Design review of the part built by this model. Coordinates are the model's own, in mm. A direction names the side the tool comes from. Give positions to 0.01 mm unless a question says otherwise; leave off trailing zeros. Order: outer loops, then holes, each group sorted by start corner. A loop starts at its lowest first (then second) coordinate and runs counter-clockwise, first axis right, second up. Notation, with made-up numbers: (12, -21.5) -> (71, -21.5) arc R18 cw to (71, -9.5) -> close; hole circle Ø7 at (6, 38). An arc over 180 degrees is marked (long way). Answer in a Markdown table with one row per item. Add a question column.
```python
from build123d import *

# Parameters (mm, degrees)
BOSS_EXTRUDE2_DEPTH      = 25
BOSS_EXTRUDE2_DEPTH_BACK = 150
SKETCH3_R                = 35
SKETCH4_R                = 35
SKETCH4_R_2              = 15
CUT_EXTRUDE1_DEPTH       = 40
CUT_EXTRUDE2_START       = -80
CUT_EXTRUDE2_DEPTH       = 80
SKETCH7_R                = 15
CUT_EXTRUDE3_DEPTH       = 164.554272338


with BuildPart() as part:
    # Sketch3 → Boss-Extrude2 (new, two sides: drawn at the far end of the back side and taken through both)
    with BuildSketch(Plane.XY.offset(-BOSS_EXTRUDE2_DEPTH_BACK)):
        Circle(SKETCH3_R)
    extrude(amount=BOSS_EXTRUDE2_DEPTH + BOSS_EXTRUDE2_DEPTH_BACK)

    # Sketch4 → Cut-Extrude1 (cut)
    with BuildSketch(Plane(origin=(0, 0, -150), x_dir=(-1, 0, 0), z_dir=(0, 0, -1))):
        Circle(SKETCH4_R)
        Circle(SKETCH4_R_2, mode=Mode.SUBTRACT)
    extrude(amount=-CUT_EXTRUDE1_DEPTH, mode=Mode.SUBTRACT)

    # Sketch5 → Cut-Extrude2 (cut)
    with BuildSketch(Plane.XY.offset(25).offset(CUT_EXTRUDE2_START)):
        with BuildLine():
            Line((-28.722813233, 20), (28.722813233, 20))
            ThreePointArc((28.722813233, 20), (0, 35), (-28.722813233, 20))
        make_face()
        with BuildLine():
            Line((-28.722813233, -20), (28.722813233, -20))
            ThreePointArc((28.722813233, -20), (0, -35), (-28.722813233, -20))
        make_face()
    extrude(amount=CUT_EXTRUDE2_DEPTH, mode=Mode.SUBTRACT)

    # Sketch7 → Cut-Extrude3 (cut, through all)
    with BuildSketch(Plane.XZ.offset(20)):
        with Locations(Location((0, 0, 0), (0, 0, 270))):
            Circle(SKETCH7_R)
    extrude(amount=-CUT_EXTRUDE3_DEPTH, mode=Mode.SUBTRACT)


solid = part.part
```
1) Clearance check with flat-ended pins moving along their axes: P1, Ø2, axis at y = -5.5, z = -25, coming from the +X side; P2, Ø7.5, axis at x = 2.5, y = -30.5, coming from the +Z side; P3, Ø1, axis at y = -19.5, z = -96, coming from the +X side. State where each tip first meets the part, or that it passes through.
2) For L1, parallel to Y at x = 0.5, z = -90; L2, parallel to Y at x = 22.5, z = -49; L3, parallel to Z at x = 30.5, y = -17, list the stretches that pass through material, from the lowest coordinate up.
3) Add section B-B, the plane z = 0. Write out the cut boundary in (x, y).
4) Mouldability with a two-part tool opening along X and no side actions: class faces 4 (the face through (0.66, -0.28, 14.985)), 5 (the face through (33.384, 10.513, -58.445)), 6 (the face through (-15, -7, -110)) as +X half, -X half, draft (parallel to the pull), parting line (faces both ways), or undercut.
5) Add section D-D, the plane y = 0. Write out the cut boundary in (x, z).
6) Machinability: for faces 1 (the face through (0, -26, -55)), 2 (the face through (14.985, 0.66, -130.28)), 3 (the face through (0, 20, -16)), which of the approach directions +Z, -Z, +X, -X, +Y, -Y give a long, thin tool a straight path to every point of the face, cutting with its end or side? Answer none if there is none.
7) Add section C-C, the plane x = -21. Write out the cut boundary in (y, z), and give its area (3 significant figures).
8) Add section A-A, the plane x = 0. Write out the cut boundary in (y, z), and give its area (3 significant figures).
Verdict:
| question | item | result |
|---|---|---|
| 1 | P1 | stops at x = 34.71 |
| 1 | P2 | stops at z = -55 |
| 1 | P3 | stops at x = 29.39 |
| 2 | L1 | y = -35 to 35 |
| 2 | L2 | y = -20 to 20 |
| 2 | L3 | z = -110 to 25 |
| 3 | outline | (-28.72, -20) -> (-15, -20) -> (-15, 20) -> (-28.72, 20) arc R35 ccw to start; (15, -20) -> (28.72, -20) arc R35 ccw to (28.72, 20) -> (15, 20) -> close |
| 4 | face 4 | undercut |
| 4 | face 5 | parting line |
| 4 | face 6 | draft |
| 5 | outline | (-35, -110) -> (-15, -110) -> (-15, -150) -> (15, -150) -> (15, -110) -> (35, -110) -> (35, 25) -> (-35, 25) -> close; hole circle Ø30 at (0, 0) |
| 6 | face 1 | +Z, +X, -X, -Y |
| 6 | face 2 | -Z |
| 6 | face 3 | +Z, +X, -X, +Y |
| 7 | outline | (-28, -110) -> (28, -110) -> (28, -55) -> (20, -55) -> (20, 25) -> (-20, 25) -> (-20, -55) -> (-28, -55) -> close |
| 7 | area | 6,280 mm2 |
| 8 | outline | (-35, -110) -> (-15, -110) -> (-15, -150) -> (15, -150) -> (15, -110) -> (35, -110) -> (35, -55) -> (20, -55) -> (20, -15) -> (-20, -15) -> (-20, -55) -> (-35, -55) -> close; (-20, 15) -> (20, 15) -> (20, 25) -> (-20, 25) -> close |
| 8 | area | 7,050 mm2 |
